Verification items for the finished model (mm, model axes). Face numbers are marked on the shaded views. A direction names the side the tool comes from. Coordinates: 2 decimals unless noted, no trailing zeros. Write each loop counter-clockwise with the first axis right and the second up, starting at its lowest first coordinate (ties: lowest second). Pieces come first, ordered by that corner, then holes. Notation, with made-up numbers: (53, 52) -> (81, 52) arc R26 ccw to (81, 91) -> close; hole circle Ø8 at (22.5, -34.5). An arc over 180 degrees is marked (long way). Answer in a Markdown table with one row per item.
```python
from build123d import *

# Parameters (mm, degrees)
F2_SIZE2 = 2.54
F2_SIZE  = 2.54


with BuildPart() as f1:
    # F0 (on Front) → F1 (revolve)
    with BuildSketch(Plane.XZ):
        Polygon((4.7625, 0), (25.4, 0), (25.4, 6.35), (20.6375, 6.35), (20.6375, 15.875), (9.525, 15.875), (9.525, 6.35), (4.7625, 6.35), align=None)
    revolve(axis=Axis((0, 0, 16.889236), (0, 0, 1)))

    # F2
    f2_edges = [f1.edges().sort_by_distance(p)[0] for p in [
        (-20.6375, 0, 15.875),
        (-25.4, 0, 0),
    ]]
    chamfer(f2_edges, length=F2_SIZE, length2=F2_SIZE2)


solid = f1.part
```
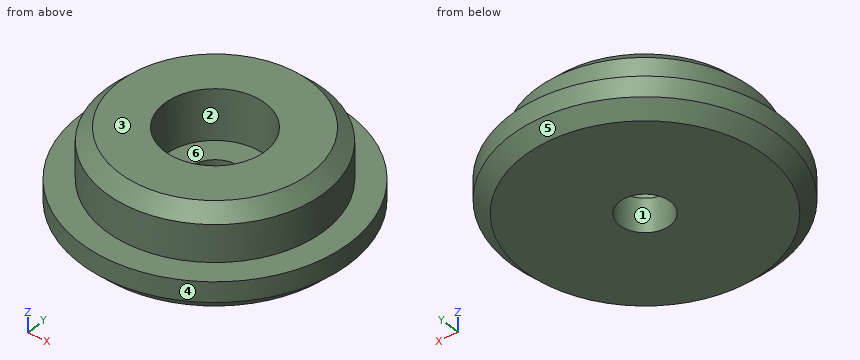
1. Section check D-D, the plane z = 4.25. Record the boundary of the cut face in (x, y) (1 decimal), plus the area to 3 significant figures.
Geometry says:
| item | result |
|---|---|
| outline | circle Ø50.8 at (0, 0); hole circle Ø9.5 at (0, 0) |
| area | 1,960 mm^2 |
2. Thickness scan on line 1 (Y direction, x = 0, z = 3); line 2 (Y direction, x = 0, z = 8.5) (1 decimal); line 3 (X direction, y = -3, z = 0.5). Record the ranges inside material, lowest first. Write a range as from..to.
Geometry says:
| item | result |
|---|---|
| line 1 | -25.4..-4.76, 4.76..25.4 |
| line 2 | -20.6..-9.5, 9.5..20.6 |
| line 3 | -23.17..-3.7, 3.7..23.17 |
3. Tool access check on the marked faces 5 and 6. Record the directions out of +Z, -Z, +X, -X, +Y, -Y that give a thin tool (end or side, any length) a straight path to the whole face; none if there is none.
Geometry says:
| item | result |
|---|---|
| face 5 | -Z |
| face 6 | +Z |
4. Depth check by flat-ended pin: P1, Ø8, axis at x = -14.5, y = 3.5, coming from the -Z side; P2, Ø9.5, axis at x = 0.5, y = -4.5, coming from the +Z side; P3, Ø4, axis at x = 6.5, z = 11, coming from the -Y side; P4, Ø3, axis at y = -15.5, z = 13, coming from the -X side. Enter the tip coordinate at first touch or a pass-through.
Geometry says:
| item | result |
|---|---|
| P1 | z = 0 |
| P2 | z = 6.35 |
| P3 | y = -20.14 |
| P4 | x = -15.16 |
5. Mould release check, pull along Y, two halves, no side actions. Record for the marked faces 1, 2, 3 and 4: released by +Y, released by -Y, zero draft, split by the parting line, or undercut.
Geometry says:
| item | result |
|---|---|
| face 1 | undercut |
| face 2 | undercut |
| face 3 | zero draft |
| face 4 | split by the parting line |
